The listing builds one solid part. Answer for the finished solid, in the listing's coordinates (mm). Face numbers are marked on the shaded views. A direction names the side the tool comes from. Round coordinates to 2 decimals unless told otherwise and drop trailing zeros. Write each loop counter-clockwise with the first axis right and the second up, starting at its lowest first coordinate (ties: lowest second). Pieces come first, ordered by that corner, then holes. Notation, with made-up numbers: (75, 25) -> (88, 25) arc R4 cw to (88, 31) -> close; hole circle Ø4 at (-12, 10.25). An arc over 180 degrees is marked (long way). Write each question's results on one line, items separated by ' | '. Start each with the question number.
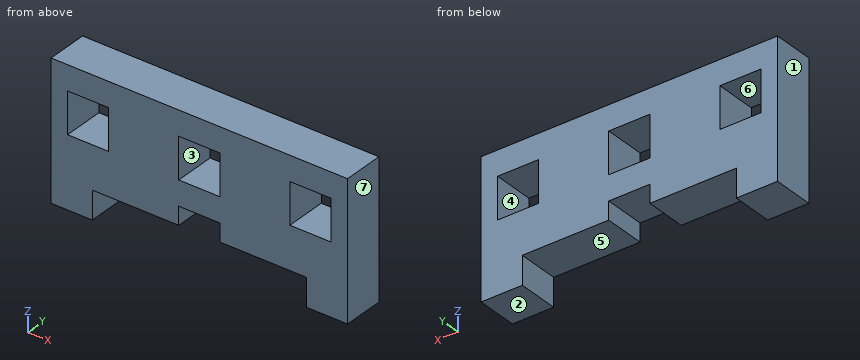
```python
from build123d import *

# Parameters (mm, degrees)
SKETCH1_W           = 6.35
SKETCH1_H           = 6.35
BOSS_EXTRUDE1_DEPTH = 6.35


with BuildPart() as part:
    # Sketch1 → Boss-Extrude1 (new body)
    with BuildSketch(Plane(origin=(0, 0, 0), x_dir=(1, 0, 0), z_dir=(0, 1, 0))):
        Polygon((-22.86, -6.985), (22.86, -6.985), (22.86, 9.757500043), (22.86, 14.102499989), (16.51, 14.102499989), (16.51, 9.757500043), (3.175, 9.757500043), (3.175, 6.985), (-3.175, 6.985), (-3.175, 9.757500043), (-16.51, 9.757500043), (-16.51, 14.102499989), (-22.86, 14.102499989), (-22.86, 9.757500043), align=None)
        Rectangle(SKETCH1_W, SKETCH1_H, mode=Mode.SUBTRACT)
        with Locations((17.145, 0)):
            Rectangle(SKETCH1_W, SKETCH1_H, mode=Mode.SUBTRACT)
        with Locations((-17.145, 0)):
            Rectangle(SKETCH1_W, SKETCH1_H, mode=Mode.SUBTRACT)
    extrude(amount=BOSS_EXTRUDE1_DEPTH)


solid = part.part
```
Q1. The part is cut by section B-B, the plane y = 1.25. Write down the section's boundary in (x, z) (1 decimal), then the cut area to 3 significant figures.
Q2. The part is cut by section A-A, the plane z = -11. Write down the section's boundary in (x, y).
Q3. For the marked faces 5, 6 and 7, determine the directions among +Z, -Z, +X, -X, +Y, -Y from which every point of the face is accessible in a straight line to the end or side of a thin tool.
Q4. Find the intervals of material crossed by line 1 (X direction, y = 3.25, z = 2.75) (3 decimals); line 2 (Z direction, x = -16, y = 4.5) (1 decimal); line 3 (Z direction, x = 17, y = 4.75) (1 decimal), in increasing order.
Q5. Determine the mould class of the marked faces 1, 2, 3 and 4 for opening direction X: pulls with the +X half, pulls with the -X half, needs draft (parallel to the pull), parting line crosses it, or undercut.
Q6. Each of these flat-tipped pins is pushed along its axis until it touches: pin 1 (3 mm diameter, centred on x = -1, y = 4, fed in from -Z) (3 decimals); pin 2 (1.9 mm diameter, centred on x = 7, y = 4.5, fed in from -Z). Where does it stop, or does it pass through?
Answers follow:
1) outline: (-22.9, -14.1) -> (-16.5, -14.1) -> (-16.5, -9.8) -> (-3.2, -9.8) -> (-3.2, -7) -> (3.2, -7) -> (3.2, -9.8) -> (16.5, -9.8) -> (16.5, -14.1) -> (22.9, -14.1) -> (22.9, 7) -> (-22.9, 7) -> close; hole (-20.3, -3.2) -> (-14, -3.2) -> (-14, 3.2) -> (-20.3, 3.2) -> close; hole (-3.2, -3.2) -> (3.2, -3.2) -> (3.2, 3.2) -> (-3.2, 3.2) -> close; hole (14, -3.2) -> (20.3, -3.2) -> (20.3, 3.2) -> (14, 3.2) -> close | area: 682 mm^2
2) outline: (-22.86, 0) -> (-16.51, 0) -> (-16.51, 6.35) -> (-22.86, 6.35) -> close; (16.51, 0) -> (22.86, 0) -> (22.86, 6.35) -> (16.51, 6.35) -> close
3) face 5: -Z, +Y, -Y | face 6: +Y, -Y | face 7: +Z, -Z, +X, +Y, -Y
4) line 1: -22.86 to -20.32, -13.97 to -3.175, 3.175 to 13.97, 20.32 to 22.86 | line 2: -9.8 to -3.2, 3.2 to 7 | line 3: -14.1 to -3.2, 3.2 to 7
5) face 1: pulls with the -X half | face 2: needs draft | face 3: undercut | face 4: undercut
6) pin 1: z = -6.985 | pin 2: z = -9.76
